Design review of the part built by this model. Coordinates are the model's own, in mm. A direction names the side the tool comes from. Coordinates: 2 decimals unless noted, no trailing zeros. Write each loop counter-clockwise with the first axis right and the second up, starting at its lowest first coordinate (ties: lowest second). Pieces come first, ordered by that corner, then holes. Notation, with made-up numbers: (78.5, 55) - (82.5, 55) arc R25 cw to (82.5, 85) - close; hole circle Ø3 at (-20.5, 10.5). An arc over 180 degrees is marked (long way). Answer as CSV lines item,"result". Start each with the question number.
Q1. Clearance check with flat-ended pins moving along their axes: pin 1 (1 mm diameter, centred on y = 2, z = -44.5, fed in from +X); pin 2 (0.8 mm diameter, centred on y = 5, z = 178.5, fed in from -X); pin 3 (1.5 mm diameter, centred on x = 0, z = 186, fed in from +Y). State where each tip first meets the part, or that it passes through.
Q2. We need section C-C (z = -33). Write out the cut boundary in (x, y).
Q3. For line 1 along Z through (x, y) = (5.5, 8.25); line 2 along X through (y, z) = (-0.75, -120.5); line 3 along Y through (x, z) = (0, -46), list the stretches that pass through material, from the lowest coordinate up. Write a range as [from, to].
Q4. Mouldability with a two-part tool opening along Z and no side actions: class faces 3 (the face through (-7, -2, 136.3)), 4 (the face through (0, 6.5, -1)), 5 (the face through (0, 0, -136.3)), 6 (the face through (-2.17, -9.76, 1.91)) as pulls with the +Z half, pulls with the -Z half, needs draft (parallel to the pull), parting line crosses it, or undercut.
Q5. We need section A-A (y = 0). Write out the cut boundary in (x, z).
Q6. Machinability: for faces 1 (the face through (-1.517, -6.834, 171.303)), 2 (the face through (0, 0, 207.3)), which of the approach directions +Z, -Z, +X, -X, +Y, -Y give a long, thin tool a straight path to every point of the face, cutting with its end or side? Answer none if there is none.
Q7. We need section B-B (z = 65). Write out the cut boundary in (x, y).
from build123d import *

# Parameters (mm, degrees)
IZIM1_R                     = 10
Y_KSEKLIK_EKSTR_ZYON1_DEPTH = 136.3
IZIM2_R                     = 7
Y_KSEKLIK_EKSTR_ZYON2_DEPTH = 71
KES_EKSTR_ZYON1_DEPTH       = 3
KES_EKSTR_ZYON2_DEPTH       = 3.5


with BuildPart() as part:
    # Çizim1 → Yükseklik-Ekstrüzyon1 (new, symmetric)
    with BuildSketch(Plane.XY):
        Circle(IZIM1_R)
    extrude(amount=Y_KSEKLIK_EKSTR_ZYON1_DEPTH, both=True)

    # Çizim2 → Yükseklik-Ekstrüzyon2 (add)
    with BuildSketch(Plane.XY.offset(136.3)):
        Circle(IZIM2_R)
    extrude(amount=Y_KSEKLIK_EKSTR_ZYON2_DEPTH)

    # Çizim3 → Kes-Ekstrüzyon1 (cut)
    with BuildSketch(Plane(origin=(0, 7, 0), x_dir=(1, 0, 0), z_dir=(0, 1, 0))):
        with BuildLine():
            Line((2.5, -155.3), (2.5, -195.3))
            ThreePointArc((2.5, -195.3), (0, -197.8), (-2.5, -195.3))
            Line((-2.5, -195.3), (-2.5, -155.3))
            ThreePointArc((-2.5, -155.3), (0, -152.8), (2.5, -155.3))
        make_face()
    extrude(amount=-KES_EKSTR_ZYON1_DEPTH, mode=Mode.SUBTRACT)

    # Çizim4 → Kes-Ekstrüzyon2 (cut)
    with BuildSketch(Plane(origin=(0, 10, 0), x_dir=(1, 0, 0), z_dir=(0, 1, 0))):
        with BuildLine():
            Line((-3, -40), (-3, 40))
            ThreePointArc((-3, 40), (0, 43), (3, 40))
            Line((3, 40), (3, -40))
            ThreePointArc((3, -40), (0, -43), (-3, -40))
        make_face()
    extrude(amount=-KES_EKSTR_ZYON2_DEPTH, mode=Mode.SUBTRACT)


solid = part.part
Results list:
1,pin 1,"stops at x = 9.89"
1,pin 2,"stops at x = -5.28"
1,pin 3,"stops at y = 4"
2,outline,"(-3, 6.5) - (-3, 9.54) arc R10 ccw (long way) to (3, 9.54) - (3, 6.5) - close"
3,line 1,"z = [-136.3, 136.3]"
3,line 2,"x = [-9.97, 9.97]"
3,line 3,"y = [-10, 10]"
4,face 3,"pulls with the +Z half"
4,face 4,"undercut"
4,face 5,"pulls with the -Z half"
4,face 6,"needs draft"
5,outline,"(-10, -136.3) - (10, -136.3) - (10, 136.3) - (7, 136.3) - (7, 207.3) - (-7, 207.3) - (-7, 136.3) - (-10, 136.3) - close"
6,face 1,"+Z"
6,face 2,"+Z, +X, -X, +Y, -Y"
7,outline,"circle Ø20 at (0, 0)"
